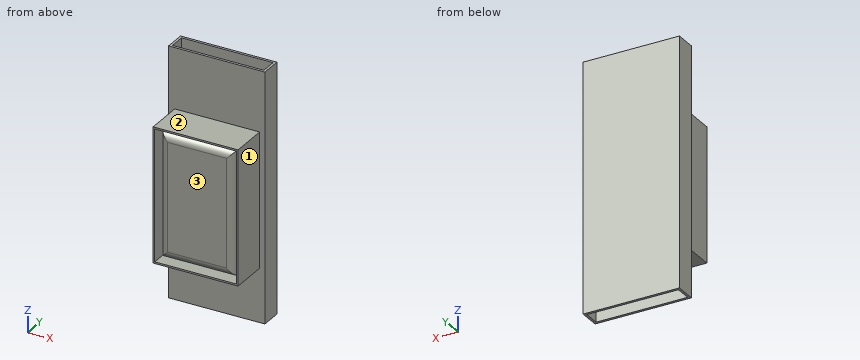
```python
from build123d import *

# Parameters (mm, degrees)
F0_W          = 590
F0_H          = 128
F1_DEPTH      = 1520
F2_W          = 560
F2_H          = 98
F3_DEPTH      = 1520.001
F4_W          = 460
F4_H          = 762
F5_DEPTH      = 215
F5_DEPTH_BACK = 128
F6_R          = 50
F7_W          = 520
F7_H          = 822
F7_W_2        = 500
F7_H_2        = 802
F8_DEPTH      = 231.234834


with BuildPart() as f1:
    # F0 (on Top) → F1 (new body)
    with BuildSketch(Plane.XY):
        Rectangle(F0_W, F0_H)
    extrude(amount=F1_DEPTH)

    # F2 (on face) → F3 (cut, through all)
    with BuildSketch(Plane.XY.offset(1520)):
        Rectangle(F2_W, F2_H)
    extrude(amount=-F3_DEPTH, mode=Mode.SUBTRACT)

    # F4 (on face) → F5 (join, two sides)
    with BuildSketch(Plane.XZ.offset(64)) as f5_sk:
        with Locations((3, 739)):
            Rectangle(F4_W, F4_H)
    extrude(amount=F5_DEPTH)
    extrude(f5_sk.sketch, amount=-F5_DEPTH_BACK)

    # F6
    f6_edges = [f1.edges().sort_by_distance(p)[0] for p in [
        (233, -279, 739),
        (-227, -279, 739),
        (3, -279, 358),
        (3, -279, 1120),
    ]]
    fillet(f6_edges, radius=F6_R)

    # F7 (on face) → F8 (join)
    with BuildSketch(Plane.XZ.offset(64)):
        with Locations((3, 739)):
            Rectangle(F7_W, F7_H)
        with Locations((3, 739)):
            Rectangle(F7_W_2, F7_H_2, mode=Mode.SUBTRACT)
    extrude(amount=F8_DEPTH)


solid = f1.part
```
The listing builds one solid part. Answer for the finished solid, in the listing's coordinates (mm). Face numbers are marked on the shaded views. Round coordinates to 2 decimals unless told otherwise and drop trailing zeros. Loops run counter-clockwise (first coordinate to the right, second up) from the corner with the lowest first, then second, coordinate; pieces in that order, holes last.
Q1. Given pin 1 Ø1 at (x, y) = (126.5, -253.5) entering from -Z; pin 2 Ø2 at (y, z) = (-225.5, 788) entering from -X; pin 3 Ø5 at (x, y) = (-207.5, 22.5) entering from +Z, each flat-ended and moving along its own axis, determine where each tip first touches the part or whether it passes through.
Q2. For a pull along Z with two mould halves and no side action, classify the marked faces 1, 2 and 3 as released by +Z, released by -Z, zero draft, split by the parting line, or undercut.
Q3. Section A-A, the plane y = -188.5 is taken. Determine the outline of the cut face in (x, z).
Q4. Section B-B, the plane z = 239.5 is taken. Determine the outline of the cut face in (x, y).
Q5. Find the intervals of material crossed by line 1 (Z direction, x = -123.5, y = -79); line 2 (X direction, y = -118, z = 808); line 3 (X direction, y = -35, z = 358.5), in increasing order.
Q6. Section C-C, the plane y = -27.5 is taken. Determine the outline of the cut face in (x, z), then the cut area to 3 significant figures.
Q7. Section D-D, the plane z = 482 is taken. Determine the outline of the cut face in (x, y).
Completed:
1. pin 1: stops at z = 328
1. pin 2: stops at x = -257
1. pin 3: stops at z = 1120
2. face 1: zero draft
2. face 2: released by +Z
2. face 3: undercut
3. outline: (-257, 328) - (263, 328) - (263, 1150) - (-257, 1150) - close; (-227, 358) - (233, 358) - (233, 1120) - (-227, 1120) - close; hole (-247, 338) - (253, 338) - (253, 1140) - (-247, 1140) - close
4. outline: (-295, -64) - (295, -64) - (295, 64) - (-295, 64) - close; hole (-280, -49) - (280, -49) - (280, 49) - (-280, 49) - close
5. line 1: z = 328 to 338, 358 to 1120, 1140 to 1150
5. line 2: x = -257 to -247, -227 to 233, 253 to 263
5. line 3: x = -295 to -280, -227 to 233, 280 to 295
6. outline: (-295, 0) - (-280, 0) - (-280, 1520) - (-295, 1520) - close; (-227, 358) - (233, 358) - (233, 1120) - (-227, 1120) - close; (280, 0) - (295, 0) - (295, 1520) - (280, 1520) - close
6. area: 396,000 mm2
7. outline: (-295, -64) - (-257, -64) - (-257, -295.23) - (-247, -295.23) - (-247, -64) - (-227, -64) - (-227, -229) arc R50 ccw to (-177, -279) - (183, -279) arc R50 ccw to (233, -229) - (233, -64) - (253, -64) - (253, -295.23) - (263, -295.23) - (263, -64) - (295, -64) - (295, 64) - (-295, 64) - close; hole (-280, -49) - (-227, -49) - (-227, 49) - (-280, 49) - close; hole (233, -49) - (280, -49) - (280, 49) - (233, 49) - close
